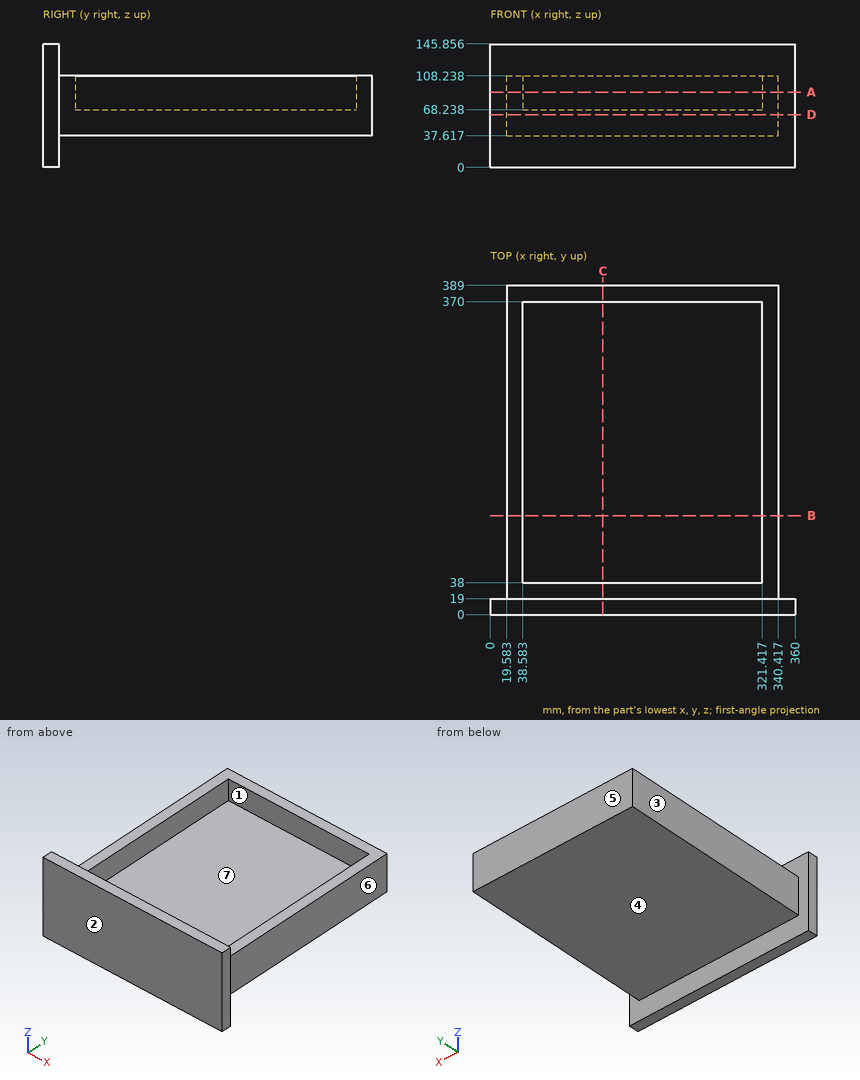
The drawing under review shows one solid part. Ordinate dimensions are in mm from its lowest x, y, z. A direction names the side the tool comes from. Round coordinates to 2 decimals unless told otherwise and drop trailing zeros. Order: outer loops, then holes, each group sorted by start corner. A loop starts at its lowest first (then second) coordinate and runs counter-clockwise, first axis right, second up. Notation, with made-up numbers: (82.25, 71.25) -> (134.25, 71.25) arc R19 cw to (134.25, 75.25) -> close; hole circle Ø10 at (-14, 57). An arc over 180 degrees is marked (long way). Use a Markdown table: item, result.
Q1. We need section D-D on z = 62.5. Write out the cut boundary in (x, y), then the cut area to 3 significant figures.
Values:
| item | result |
|---|---|
| outline | (0, 0) -> (360, 0) -> (360, 19) -> (340.42, 19) -> (340.42, 389) -> (19.58, 389) -> (19.58, 19) -> (0, 19) -> close |
| area | 126,000 mm^2 |
Q2. We need section B-B on y = 117. Write out the cut boundary in (x, z), then the cut area to 3 significant figures.
Values:
| item | result |
|---|---|
| outline | (19.58, 37.62) -> (340.42, 37.62) -> (340.42, 108.24) -> (321.42, 108.24) -> (321.42, 68.24) -> (38.58, 68.24) -> (38.58, 108.24) -> (19.58, 108.24) -> close |
| area | 11,300 mm^2 |
Q3. Clearance check with flat-ended pins moving along their axes: P1, Ø20, axis at y = 132.5, z = 86, coming from the +X side; P2, Ø2, axis at y = 291.5, z = 38, coming from the -X side; P3, Ø1.5, axis at x = 234.5, y = 82, coming from the -Z side; P4, Ø8, axis at x = 233.5, z = 101, coming from the -Y side. State where each tip first meets the part, or that it passes through.
Values:
| item | result |
|---|---|
| P1 | stops at x = 340.42 |
| P2 | stops at x = 19.58 |
| P3 | stops at z = 37.62 |
| P4 | stops at y = 0 |
Q4. We need section A-A on z = 89. Write out the cut boundary in (x, y).
Values:
| item | result |
|---|---|
| outline | (0, 0) -> (360, 0) -> (360, 19) -> (340.42, 19) -> (340.42, 389) -> (19.58, 389) -> (19.58, 19) -> (0, 19) -> close; hole (38.58, 38) -> (321.42, 38) -> (321.42, 370) -> (38.58, 370) -> close |
Q5. For line 1 (Y direction, x = 87.5, z = 69); line 2 (X direction, y = 181, z = 82.5); line 3 (Z direction, x = 304, y = 138.5), list the stretches that pass through material, from the lowest coordinate up.
Values:
| item | result |
|---|---|
| line 1 | y = 0 to 38, 370 to 389 |
| line 2 | x = 19.58 to 38.58, 321.42 to 340.42 |
| line 3 | z = 37.62 to 68.24 |
Q6. Mouldability with a two-part tool opening along Y and no side actions: class the marked faces 1, 2 and 3 as +Y half, -Y half, draft (parallel to the pull), parting line (faces both ways), or undercut.
Values:
| item | result |
|---|---|
| face 1 | undercut |
| face 2 | -Y half |
| face 3 | draft |
Q7. Tool access review of the marked faces 4, 5, 6 and 7: name each direction out of +Z, -Z, +X, -X, +Y, -Y from which nothing blocks a thin tool from reaching the whole face with its end or side.
Values:
| item | result |
|---|---|
| face 4 | -Z, +X, -X, +Y |
| face 5 | +Z, -Z, +X, -X, +Y |
| face 6 | +Z, -Z, +X, +Y |
| face 7 | +Z |
Q8. We need section C-C on x = 133. Write out the cut boundary in (y, z) (1 decimal).
Values:
| item | result |
|---|---|
| outline | (0, 0) -> (19, 0) -> (19, 37.6) -> (389, 37.6) -> (389, 108.2) -> (370, 108.2) -> (370, 68.2) -> (38, 68.2) -> (38, 108.2) -> (19, 108.2) -> (19, 145.9) -> (0, 145.9) -> close |
